Check sheet for the drawn part. Datum: minimum x, y, z corner. Units: mm. Round coordinates to 2 decimals unless told otherwise and drop trailing zeros. Write each loop counter-clockwise with the first axis right and the second up, starting at its lowest first coordinate (ties: lowest second). Pieces come first, ordered by that corner, then holes. Notation, with made-up numbers: (20, 72) -> (71, 72) arc R29 ccw to (71, 95) -> close; hole circle Ø7 at (20, 42). An arc over 180 degrees is marked (long way). Use a Markdown table: item, result.
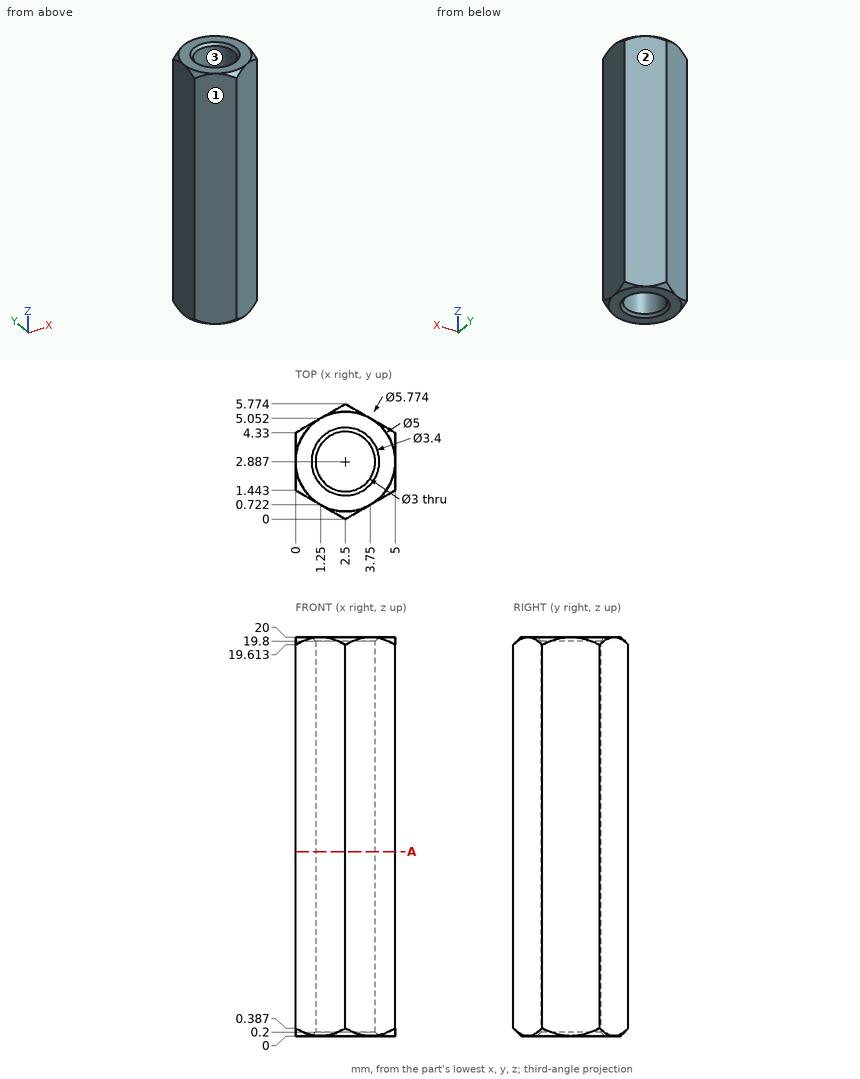
(1) Release check for a two-part mould opening along Y. For the marked faces 1, 2 and 3 record: +Y half, -Y half, draft (parallel to the pull), parting line (faces both ways), or undercut.
A:
| item | result |
|---|---|
| face 1 | -Y half |
| face 2 | +Y half |
| face 3 | undercut |
(2) Gauge pin test, flat ends, axial feed: pin 1 Ø3 at (x, z) = (1.5, 2.5) entering from +Y; pin 2 Ø1.5 at (x, z) = (0.5, 16.5) entering from -Y. Record the tip position at first contact, or that the pin passes through.
A:
| item | result |
|---|---|
| pin 1 | stops at y = 5.77 |
| pin 2 | stops at y = 0.72 |
(3) Section check A-A on z = 9.25. Record the cut outline in (x, y).
A:
| item | result |
|---|---|
| outline | (0, 1.44) -> (2.5, 0) -> (5, 1.44) -> (5, 4.33) -> (2.5, 5.77) -> (0, 4.33) -> close; hole circle Ø3 at (2.5, 2.89) |
(4) Thickness scan on line 1 (X direction, y = 2.05, z = 7.75) (1 decimal); line 2 (X direction, y = 2.85, z = 7); line 3 (Y direction, x = 2.7, z = 13.75) (1 decimal). Record the ranges inside material, lowest first.
A:
| item | result |
|---|---|
| line 1 | x = 0 to 1.3, 3.7 to 5 |
| line 2 | x = 0 to 1, 4 to 5 |
| line 3 | y = 0.1 to 1.4, 4.4 to 5.7 |
